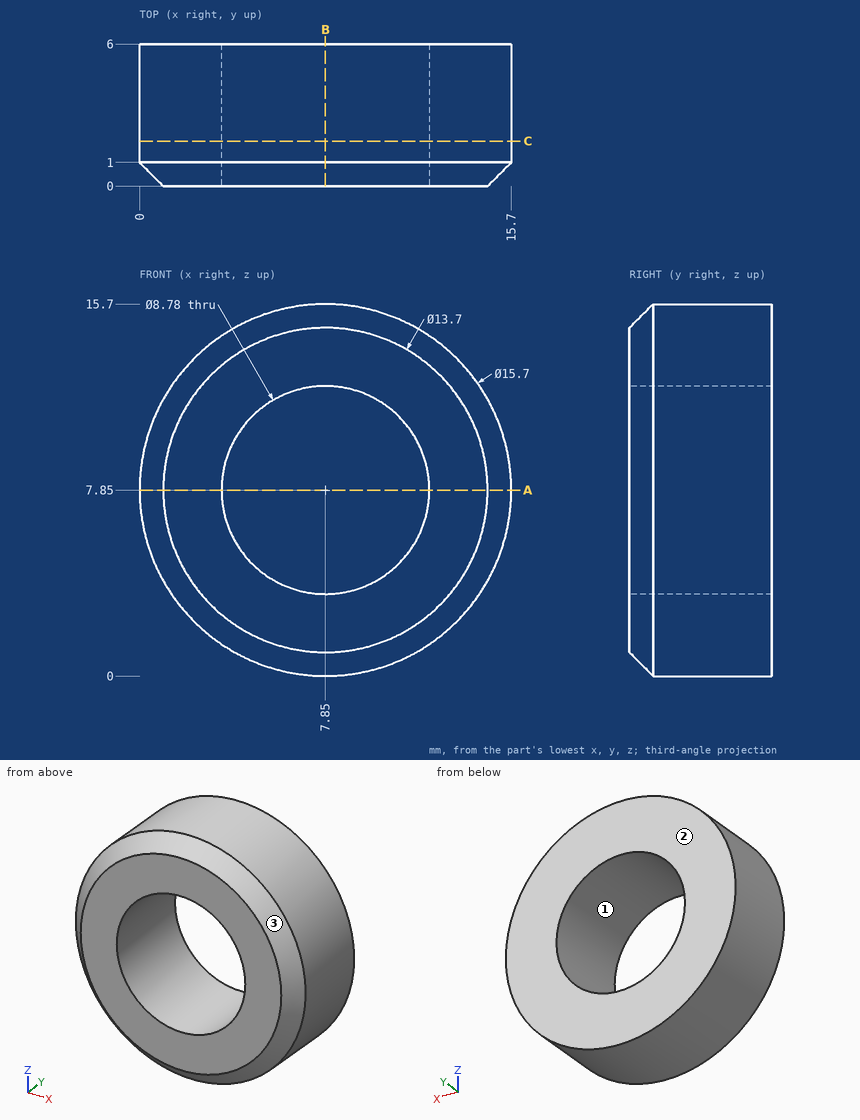
Drawing for the job (mm, zero at the part's lowest x, y, z). Round coordinates to 2 decimals unless told otherwise and drop trailing zeros. Loops run counter-clockwise (first coordinate to the right, second up) from the corner with the lowest first, then second, coordinate; pieces in that order, holes last. Notation, with made-up numbers: (-33.5, -13) - (-9.5, -13) arc R13 cw to (-9.5, -8) - close; hole circle Ø5 at (27.5, -22.5). An arc over 180 degrees is marked (long way). Write each question's results on one line, items separated by ' | '.
(1) Pin check, flat tips, straight feed: pin 1 (1.5 mm diameter, centred on y = 2, z = 3, fed in from -X); pin 2 (1.5 mm diameter, centred on y = 2.5, z = 5, fed in from +X); pin 3 (1.5 mm diameter, centred on y = 4.5, z = 5.5, fed in from -X). Stop position of each tip, or through.
Answer below:
pin 1: stops at x = 1.16 | pin 2: stops at x = 15.41 | pin 3: stops at x = 0.16
(2) Wall check: L1, parallel to Z at x = 7.85, y = 3; L2, parallel to X at y = 5.15, z = 11.5; L3, parallel to X at y = 3.8, z = 4.5. Give the ranges that are in metal, low to high.
Answer below:
L1: z = 0 to 3.46, 12.24 to 15.7 | L2: x = 0.9 to 5.41, 10.29 to 14.8 | L3: x = 0.75 to 5.01, 10.69 to 14.95
(3) Mould opens along X. For the marked faces 1, 2 and 3 say: released by +X, released by -X, zero draft, split by the parting line, or undercut.
Answer below:
face 1: undercut | face 2: zero draft | face 3: split by the parting line
(4) Saw through at B-B, the plane x = 7.85. List the corners of the cut face in (y, z), then the cut area to 3 significant figures.
Answer below:
outline: (0, 1) - (1, 0) - (6, 0) - (6, 3.46) - (0, 3.46) - close; (0, 12.24) - (6, 12.24) - (6, 15.7) - (1, 15.7) - (0, 14.7) - close | area: 40.5 mm^2
(5) Saw through at A-A, the plane z = 7.85. List the corners of the cut face in (x, y).
Answer below:
outline: (0, 1) - (1, 0) - (3.46, 0) - (3.46, 6) - (0, 6) - close; (12.24, 0) - (14.7, 0) - (15.7, 1) - (15.7, 6) - (12.24, 6) - close
(6) Saw through at C-C, the plane y = 1.9. List the corners of the cut face in (x, z).
Answer below:
outline: circle Ø15.7 at (7.85, 7.85); hole circle Ø8.78 at (7.85, 7.85)
